Part model, mm, in its own coordinate system. Round coordinates to 2 decimals unless told otherwise and drop trailing zeros. Write each loop counter-clockwise with the first axis right and the second up, starting at its lowest first coordinate (ties: lowest second). Pieces come first, ordered by that corner, then holes.
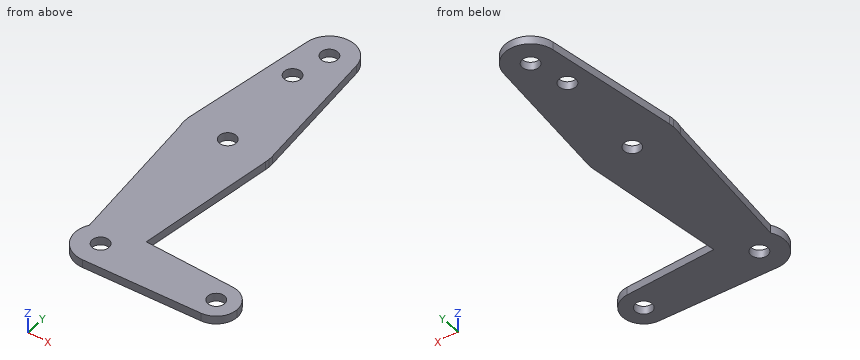
```python
from build123d import *

# Parameters (mm, degrees)
F0_R     = 3.175
F1_DEPTH = 3.048


with BuildPart() as f1:
    # F0 (on Top) → F1 (new body)
    with BuildSketch(Plane.XY):
        with BuildLine():
            ThreePointArc((15.750488268, 1.9843750453), (-2.28e-08, 15.875), (-15.7504882737, 1.984375))
            ThreePointArc((-15.7504882737, 1.984375), (-15.8438414904, 0.9941387366), (-15.875, 0))
            Line((-15.875, 0), (-15.3276351094, -4.1327021368))
            ThreePointArc((-15.3276351094, -4.1327021368), (1.2939167116, -15.8221807771), (15.7954255641, -1.5875))
            ThreePointArc((15.7954255641, -1.5875), (15.8550939106, -0.7947465541), (15.875, 0))
            ThreePointArc((15.875, 0), (15.843841489, 0.9941387594), (15.750488268, 1.9843750453))
        make_face()
        Circle(F0_R, mode=Mode.SUBTRACT)
        with BuildLine():
            Line((-9.4502929642, 51.990625), (-15.7504882737, 1.984375))
            ThreePointArc((-15.7504882737, 1.984375), (-2.28e-08, 15.875), (15.750488268, 1.9843750453))
            Line((15.750488268, 1.9843750453), (9.4502929642, 51.990625))
            ThreePointArc((9.4502929642, 51.990625), (9.5063048942, 51.396483242), (9.525, 50.8))
            ThreePointArc((9.525, 50.8), (-0.596483242, 41.2936951058), (-9.4502929642, 51.990625))
        make_face()
        with Locations((-3.175, 36.5252)):
            Circle(F0_R, mode=Mode.SUBTRACT)
        with BuildLine():
            Line((-15.3276351094, -4.1327021368), (-15.875, 0))
            ThreePointArc((-15.875, 0), (-15.7375638579, -2.0843965119), (-15.3276351094, -4.1327021368))
        make_face()
        with BuildLine():
            ThreePointArc((9.4502929642, 51.990625), (0, 60.325), (-9.4502929642, 51.990625))
            ThreePointArc((-9.4502929642, 51.990625), (-0.596483242, 41.2936951058), (9.525, 50.8))
            ThreePointArc((9.525, 50.8), (9.5063048942, 51.396483242), (9.4502929642, 51.990625))
        make_face()
        with Locations((0, 50.8)):
            Circle(F0_R, mode=Mode.SUBTRACT)
        with BuildLine():
            ThreePointArc((15.7954255641, -1.5875), (1.2939167116, -15.8221807771), (-15.3276351094, -4.1327021368))
            Line((-15.3276351094, -4.1327021368), (-8.123344071, -58.5263789745))
            ThreePointArc((-8.123344071, -58.5263789745), (-4.506590709, -55.1085600055), (0.3401785714, -53.9810765556))
            Line((0.3401785714, -53.9810765556), (10.4932062399, -54.3439161633))
            Line((10.4932062399, -54.3439161633), (15.7954255641, -1.5875))
        make_face()
        with BuildLine():
            ThreePointArc((0.3401785714, -53.9810765556), (-4.506590709, -55.1085600055), (-8.123344071, -58.5263789745))
            ThreePointArc((-8.123344071, -58.5263789745), (-8.2251369351, -68.3034099762), (0.3401785714, -73.0189234444))
            ThreePointArc((0.3401785714, -73.0189234444), (6.5147068085, -70.448684782), (9.4772553384, -64.4525))
            ThreePointArc((9.4772553384, -64.4525), (9.5130563464, -63.9768479324), (9.525, -63.5))
            ThreePointArc((9.525, -63.5), (6.8544082857, -56.8861726622), (0.3401785714, -53.9810765556))
        make_face()
        with Locations((0, -63.5)):
            Circle(F0_R, mode=Mode.SUBTRACT)
        with BuildLine():
            Line((44.7334821429, -55.5675637964), (10.4932062399, -54.3439161633))
            Line((10.4932062399, -54.3439161633), (9.4772553384, -64.4525))
            ThreePointArc((9.4772553384, -64.4525), (6.5147068085, -70.448684782), (0.3401785714, -73.0189234444))
            Line((0.3401785714, -73.0189234444), (44.7334821429, -71.4324362036))
            ThreePointArc((44.7334821429, -71.4324362036), (36.5125, -63.5), (44.7334821429, -55.5675637964))
        make_face()
        with BuildLine():
            Line((9.4772553384, -64.4525), (10.4932062399, -54.3439161633))
            Line((10.4932062399, -54.3439161633), (0.3401785714, -53.9810765556))
            ThreePointArc((0.3401785714, -53.9810765556), (6.8544082857, -56.8861726622), (9.525, -63.5))
            ThreePointArc((9.525, -63.5), (9.5130563464, -63.9768479324), (9.4772553384, -64.4525))
        make_face()
        with BuildLine():
            ThreePointArc((52.3875, -63.5), (50.1620069047, -57.9884772185), (44.7334821429, -55.5675637964))
            ThreePointArc((44.7334821429, -55.5675637964), (36.5125, -63.5), (44.7334821429, -71.4324362036))
            ThreePointArc((44.7334821429, -71.4324362036), (50.1620069047, -69.0115227815), (52.3875, -63.5))
        make_face()
        with Locations((44.45, -63.5)):
            Circle(F0_R, mode=Mode.SUBTRACT)
    extrude(amount=F1_DEPTH)


solid = f1.part
```
Q1. Cut at C-C on y = -23. Write the cut outline in (x, z).
Values follow:
outline: (-12.83, 0) - (13.64, 0) - (13.64, 3.05) - (-12.83, 3.05) - close
Q2. Drop flat-ended pins along their axis: pin 1 (1 mm diameter, centred on x = 7.5, z = 1.5, fed in from +Y); pin 2 (6 mm diameter, centred on x = 16.5, y = 31, fed in from +Z). Give the stop position or say it passes through.
Values follow:
pin 1: stops at y = 57.26
pin 2: passes through
Q3. Cut at A-A on z = 1.55. State how many separate pieces and enclosed holes the cut face has, plus the area to 3 significant figures.
Values follow:
separate pieces: 1
enclosed holes: 5
area: 3,700 mm2
Q4. Cut at B-B on x = 20.5. Write the cut outline in (y, z), plus the area to 3 significant figures.
Values follow:
outline: (-72.3, 0) - (-54.7, 0) - (-54.7, 3.05) - (-72.3, 3.05) - close
area: 53.6 mm2
Q5. Wall check: L1, parallel to Y at x = -1.5, z = 2.65; L2, parallel to Y at x = 44.45, z = 1.1 (3 decimals); L3, parallel to Y at x = 36, z = 1.65. Give the ranges that are in metal, low to high.
Values follow:
L1: y = -72.91 to -66.3, -60.7 to -2.8, 2.8 to 33.83, 39.22 to 48, 53.6 to 60.21
L2: y = -71.443 to -66.675, -60.325 to -55.557
L3: y = -71.74 to -55.26
